Verification items for the finished model (mm, model axes). Give positions to 0.01 mm unless a question says otherwise; leave off trailing zeros. Write each loop counter-clockwise with the first axis right and the second up, starting at its lowest first coordinate (ties: lowest second). Pieces come first, ordered by that corner, then holes. Notation, with made-up numbers: M -13,3 L 41,3 A8 cw 41,9 Z; hole C -37,-21 d9. An arc over 180 degrees is marked long. Answer as a JSON object with one key per item and string values.
```python
from build123d import *

# Parameters (mm, degrees)
F1_DEPTH = 6.2
F2_R     = 1


with BuildPart() as f1:
    # F0 (on Top) → F1 (new body)
    with BuildSketch(Plane.XY):
        with BuildLine():
            ThreePointArc((20.897846779, -15.3), (0, 25.9), (-20.897846779, -15.3))
            Line((-20.897846779, -15.3), (20.897846779, -15.3))
        make_face()
    extrude(amount=F1_DEPTH)

    # F2
    f2_edges = [f1.edges().sort_by_distance(p)[0] for p in [
        (-20.897847, -15.3, 3.1),
        (0, 25.9, 6.2),
        (0, -15.3, 6.2),
        (20.897847, -15.3, 3.1),
    ]]
    fillet(f2_edges, radius=F2_R)


solid = f1.part
```
1) Thickness scan on L1, parallel to Z at x = -15, y = 20; L2, parallel to Y at x = 23.5, z = 0.75; L3, parallel to X at y = -7.5, z = 3. Record the ranges inside material, lowest first.
Completed:
{"L1": "z = 0 to 6.19", "L2": "y = -10.89 to 10.89", "L3": "x = -24.79 to 24.79"}
2) Section check A-A on z = 1.75. Record the boundary of the cut face in (x, y), and give its area (3 significant figures).
Completed:
{"outline": "M -21.2,-14.87 A1 ccw -20.38,-15.3 L 20.38,-15.3 A1 ccw 21.2,-14.87 A25.9 ccw long Z", "area": "1,800 mm2"}
3) Go/stop test with flat-tipped pins: pin 1 (1.5 mm diameter, centred on x = 4, z = 1, fed in from +Y); pin 2 (2 mm diameter, centred on y = -8.5, z = 1.5, fed in from -X). Record where each tip stops, or that it passes through.
Completed:
{"pin 1": "stops at y = 25.7", "pin 2": "stops at x = -24.79"}
